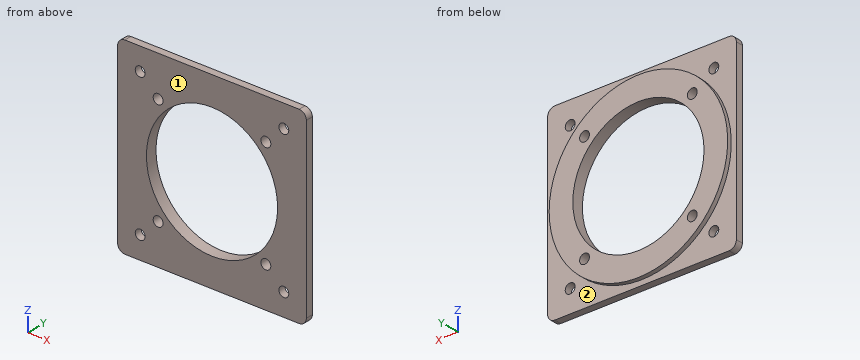
Autodesk Inventor part; units mm, degrees
ref_plane "YZ Plane" through (0, 0, 0) normal (1, 0, 0) x (0, 1, 0)
ref_plane "XZ Plane" through (0, 0, 0) normal (0, 1, 0) x (-1, 0, 0)
ref_plane "XY Plane" through (0, 0, 0) normal (0, 0, 1) x (1, 0, 0)
sketch "Sketch1" plane through (0, 0, 0) normal (0, 1, 0) x (-1, 0, 0)
  line L0 (41.275, 41.275) -> (-41.275, 41.275)
  line L1 (-41.275, 41.275) -> (-41.275, -41.275)
  line L2 (-41.275, -41.275) -> (41.275, -41.275)
  line L3 (41.275, -41.275) -> (41.275, 41.275)
  circle A0 centre (0, 0) radius 44.45 construction
  circle A1 centre (0, 0) radius 39.6875
  line L4 (-41.275, 41.275) -> (41.275, -41.275) construction
  line L5 (41.275, 41.275) -> (-41.275, -41.275) construction
  circle A2 centre (31.4309, 31.4309) radius 2.159
  circle A3 centre (31.4309, -31.4309) radius 2.159
  circle A4 centre (-31.4309, 31.4309) radius 2.159
  circle A5 centre (-31.4309, -31.4309) radius 2.159
  point P0 (0, 0)
  point P1 (0, 0)
  point P2 (0, 0)
  dimension "d0" = 82.55
  dimension "d1" = 82.55
  dimension "d2" = 88.9
  dimension "d3" = 79.375
  dimension "d4" = 4.318
  dimension "d5" = 4.318
  dimension "d6" = 4.318
  dimension "d7" = 4.318
extrude "Extrusion1" add sketch "Sketch1" along normal blind 3.175 contours L3 L2 L1 L0 | A1
sketch "Sketch2" plane through (0, 3.175, 0) normal (0, 1, 0) x (1, 0, 0)
  circle A0 centre (0, 0) radius 39.0525
  circle A1 centre (0, 0) radius 39.6875 construction
  point P0 (0, 0)
  dimension "d10" = 78.105
  dimension "d17" = 79.375
extrude "Extrusion2" add sketch "Sketch2" along normal blind 1.905
fillet "Fillet1" radius 3.175 1 edges at (41.275, 1.5875, 41.275)
fillet "Fillet2" radius 3.175 1 edges at (-41.275, 1.5875, 41.275)
fillet "Fillet3" radius 3.175 1 edges at (41.275, 1.5875, -41.275)
fillet "Fillet4" radius 3.175 1 edges at (-41.275, 1.5875, -41.275)
sketch "Sketch3" plane through (0, 5.08, 0) normal (0, 1, 0) x (1, 0, 0)
  line L0 (-30.1625, -30.1625) -> (30.1625, -30.1625) construction
  line L1 (30.1625, -30.1625) -> (30.1625, 30.1625) construction
  line L2 (30.1625, 30.1625) -> (-30.1625, 30.1625) construction
  line L3 (-30.1625, 30.1625) -> (-30.1625, -30.1625) construction
  line L4 (-30.1625, -30.1625) -> (30.1625, 30.1625) construction
  line L5 (30.1625, -30.1625) -> (-30.1625, 30.1625) construction
  circle A0 centre (0, 0) radius 33.3375 construction
  circle A1 centre (23.5732, 23.5732) radius 2.159
  circle A2 centre (23.5732, -23.5732) radius 2.159
  circle A3 centre (-23.5732, -23.5732) radius 2.159
  circle A4 centre (-23.5732, 23.5732) radius 2.159
  circle A5 centre (0, 0) radius 28.702
  dimension "d18" = 60.325
  dimension "d19" = 60.325
  dimension "d20" = 66.675
  dimension "d21" = 4.318
  dimension "d22" = 4.318
  dimension "d23" = 4.318
  dimension "d24" = 4.318
  dimension "d25" = 57.404
extrude "Extrusion3" cut sketch "Sketch3" against normal through all
properties part number "3-125-to-2-25-instrument-adapter"
Work out the finished part from the listing and answer in its coordinate system (mm). Face numbers are marked on the shaded views. A direction names the side the tool comes from. Round coordinates to 2 decimals unless told otherwise and drop trailing zeros. Write each loop counter-clockwise with the first axis right and the second up, starting at its lowest first coordinate (ties: lowest second). Pieces come first, ordered by that corner, then holes.
1) Flat-ended cylindrical pins translate along their axes: P1, Ø5, axis at x = -24.5, z = -28, coming from the -Y side; P2, Ø3.5, axis at x = -23.57, z = -23.57, coming from the +Y side; P3, Ø5.5, axis at x = -31.43, z = 31.43, coming from the +Y side (3 decimals); P4, Ø1.5, axis at x = 12.5, y = 4.5, coming from the +Z side. Find the tip coordinate at first contact, or state that the pin passes through.
2) Consider probe 1 along Z at (x, y) = (0, 2.35) (3 decimals); probe 2 along Z at (x, y) = (25, 2.45) (3 decimals); probe 3 along Z at (x, y) = (0, 3.7). Determine where each line is inside the solid, lowest interval first.
3) A cutting plane is placed at C-C on y = 1.3. Give the number of separate pieces and of enclosed holes in the cut face, and give its area (3 significant figures).
4) A cutting plane is placed at D-D on x = -31. Determine the outline of the cut face in (y, z) (3 decimals).
5) A cutting plane is placed at A-A on x = 0. Determine the outline of the cut face in (y, z) (1 decimal).
6) Which of the six approach directions +Z, -Z, +X, -X, +Y, -Y give full straight-line access (tool end or side, diameter ignored) to the marked faces 1 and 2?
7) A cutting plane is placed at B-B on z = 0. Determine the outline of the cut face in (x, y) (1 decimal).
Entries:
1. P1: stops at y = 0
1. P2: passes through
1. P3: stops at y = 3.175
1. P4: stops at z = 37.24
2. probe 1: z = -41.275 to -28.702, 28.702 to 41.275
2. probe 2: z = -41.275 to -25.194, -21.953 to -14.1, 14.1 to 21.953, 25.194 to 41.275
2. probe 3: z = -39.05 to -28.7, 28.7 to 39.05
3. separate pieces: 1
3. enclosed holes: 9
3. area: 4,100 mm2
4. outline: (0, -41.275) - (3.175, -41.275) - (3.175, -33.546) - (0, -33.546) - close; (0, -29.315) - (3.175, -29.315) - (3.175, -23.751) - (5.08, -23.751) - (5.08, 23.751) - (3.175, 23.751) - (3.175, 29.315) - (0, 29.315) - close; (0, 33.546) - (3.175, 33.546) - (3.175, 41.275) - (0, 41.275) - close
5. outline: (0, -41.3) - (3.2, -41.3) - (3.2, -39.1) - (5.1, -39.1) - (5.1, -28.7) - (0, -28.7) - close; (0, 28.7) - (5.1, 28.7) - (5.1, 39.1) - (3.2, 39.1) - (3.2, 41.3) - (0, 41.3) - close
6. face 1: +Z, -Z, +X, -X, -Y
6. face 2: +Y
7. outline: (-41.3, 0) - (-28.7, 0) - (-28.7, 5.1) - (-39.1, 5.1) - (-39.1, 3.2) - (-41.3, 3.2) - close; (28.7, 0) - (41.3, 0) - (41.3, 3.2) - (39.1, 3.2) - (39.1, 5.1) - (28.7, 5.1) - close
